The model under review builds one solid part; all positions refer to its coordinate system, in mm. A direction names the side the tool comes from. Coordinates: 2 decimals unless noted, no trailing zeros. Order: outer loops, then holes, each group sorted by start corner. A loop starts at its lowest first (then second) coordinate and runs counter-clockwise, first axis right, second up. Notation, with made-up numbers: M -20.75,45.25 L -7.75,45.25 A25 cw -7.75,65.25 Z; hole C 15,70 d3. An arc over 180 degrees is marked long. Write each question's results on one line, items separated by ' | '.
from build123d import *

# Parameters (mm, degrees)
F0_W     = 266.7
F0_H     = 15.875
F1_DEPTH = 188.9125
F2_R     = 15.875
F3_SIZE  = 7.62


with BuildPart() as f1:
    # F0 (on Front) → F1 (new body, symmetric)
    with BuildSketch(Plane.XZ):
        Rectangle(F0_W, F0_H)
        Polygon((133.35, 23.8125), (133.35, 7.9375), (133.35, -7.9375), (133.35, -42.8625), (142.875, -42.8625), (142.875, 23.8125), align=None)
        Polygon((-133.35, -7.9375), (-133.35, 7.9375), (-133.35, 23.8125), (-142.875, 23.8125), (-142.875, -42.8625), (-133.35, -42.8625), align=None)
    extrude(amount=F1_DEPTH, both=True)

    # F2
    f2_edges = [f1.edges().sort_by_distance(p)[0] for p in [
        (-138.1125, -188.9125, 23.8125),
        (-138.1125, 188.9125, 23.8125),
        (138.1125, 188.9125, 23.8125),
        (138.1125, -188.9125, 23.8125),
    ]]
    fillet(f2_edges, radius=F2_R)

    # F3
    f3_edges = [f1.edges().sort_by_distance(p)[0] for p in [
        (0, -188.9125, 7.9375),
        (0, 188.9125, 7.9375),
    ]]
    chamfer(f3_edges, length=F3_SIZE)


solid = f1.part
1) Take a section at D-D on z = 16.5. State the section outline as (x, y) points (3 decimals), plus the area to 3 significant figures.
Solutions:
outline: M -142.875,-186.405 L -133.35,-186.405 L -133.35,186.405 L -142.875,186.405 Z; M 133.35,-186.405 L 142.875,-186.405 L 142.875,186.405 L 133.35,186.405 Z | area: 7,100 mm2
2) For faces 1 (the flat face through (-2, -3, -7.938)), 2 (the flat face through (-1.87, 185.05, 4.18)), 3 (the flat face through (-2, -3, 7.938)), list the 3-axis set-ups (+Z, -Z, +X, -X, +Y, -Y) from which the entire face can be reached by the end or side of a thin tool; tool diameter is ignored.
Solutions:
face 1: -Z, +Y, -Y | face 2: +Z, +Y | face 3: +Z, +Y, -Y
3) To check wall thickness, follow line 1 along X through (y, z) = (-52.5, -12) (3 decimals); line 2 along Z through (x, y) = (129, -84.5); line 3 along Y through (x, z) = (102.5, 6.5). State the ranges of each line that lie inside material, in increasing order.
Solutions:
line 1: -142.875 to -133.35, 133.35 to 142.875 | line 2: -7.94 to 7.94 | line 3: -182.73 to 182.73
4) For pin 1 (5 mm diameter, centred on x = -27, y = 84, fed in from +Z); pin 2 (5 mm diameter, centred on x = -38, y = -105, fed in from -Z), all flat-tipped, find the tip position at first contact; note any pin that passes through.
Solutions:
pin 1: z = 7.94 | pin 2: z = -7.94
5) Take a section at C-C on x = 14.5. State the section outline as (y, z) points.
Solutions:
outline: M -188.91,-7.94 L 188.91,-7.94 L 188.91,0.32 L 181.29,7.94 L -181.29,7.94 L -188.91,0.32 Z
6) The part is to be moulded in two halves that separate along X. For faces 4 (the flat face through (-138, -3, -42.862)), 5 (the flat face through (-1.87, -185.05, 4.18)), 6 (the flat face through (-142.875, -3, -9)), say which applies: pulls with the +X half, pulls with the -X half, needs draft (parallel to the pull), parting line crosses it, or undercut.
Solutions:
face 4: needs draft | face 5: undercut | face 6: pulls with the -X half
